Autodesk Inventor part; units mm, degrees
ref_plane "YZ Plane" through (0, 0, 0) normal (1, 0, 0) x (0, 1, 0)
ref_plane "XZ Plane" through (0, 0, 0) normal (0, 1, 0) x (-1, 0, 0)
ref_plane "XY Plane" through (0, 0, 0) normal (0, 0, 1) x (1, 0, 0)
sketch "Sketch1" plane through (0, 0, 0) normal (0, 1, 0) x (-1, 0, 0)
  line L0 (0, 0) -> (25.4, 0)
  line L1 (25.4, 0) -> (25.4, -10)
  line L2 (25.4, -10) -> (0, -10)
  line L3 (0, -10) -> (0, 0)
  line L4 (25.4, -5) -> (19.05, -5)
  line L5 (19.05, -5) -> (6.35, -5)
  dimension "d0" = 25.4
  dimension "d1" = 10
  dimension "d4" = 6.35
  dimension "d5" = 12.7
extrude "Extrusion1" add sketch "Sketch1" along normal blind 4.445
hole "Hole1" at (-6.35, 0, -5) at (-19.05, 0, -5) direction (0, 1, 0) diameter 10.795 depth 3.175
sketch "Sketch2" plane through (0, 0, 0) normal (0, -1, 0) x (1, 0, 0)
  line L0 (-25.4, 0) -> (0, 0)
  line L1 (0, -10) -> (-25.4, -10)
  line L2 (0, 0) -> (-0.635, 0)
  line L3 (-0.635, 0) -> (-0.635, -10)
  line L4 (-0.635, -10) -> (0, -10)
  line L5 (0, -10) -> (0, 0)
  line L6 (-17.017, 0) -> (-8.383, 0)
  line L7 (-12.7, 0) -> (-12.0585, 0)
  line L8 (-12.0585, 0) -> (-12.0585, -10)
  line L9 (-12.0585, -10) -> (-12.7, -10)
  line L10 (-12.7, -10) -> (-12.7, 0)
  line L11 (-12.7, -10) -> (-13.3295, -10)
  line L12 (-13.3295, -10) -> (-13.3295, 0)
  line L13 (-13.3295, 0) -> (-12.7, 0)
  line L14 (-12.7, 0) -> (-12.7, -10)
  line L15 (-25.4, -10) -> (-25.4, 0)
  line L16 (-25.4, 0) -> (-21.083, 0)
  line L17 (-25.4, -10) -> (-24.765, -10)
  line L18 (-24.765, -10) -> (-24.765, 0)
  line L19 (-24.765, 0) -> (-25.4, 0)
  line L20 (-25.4, 0) -> (-25.4, -10)
  point P0 (-24.765, 0)
  dimension "d13" = 0.635
  dimension "d14" = 0.635
sketch "Sketch3" plane through (0, 0, 0) normal (1, 0, 0) x (0, 0, -1)
  line L0 (0, 4.445) -> (10, 4.445)
  line L1 (5, 4.445) -> (9.445, 0)
  line L2 (10, 0) -> (0, 0)
  line L3 (5, 4.445) -> (11.2862, 4.445) construction
  dimension "d15" = 45
extrude "Extrusion2" add sketch "Sketch2" along normal blind 25.4 contours L0 L18 L1 L15 | L12 L0 L10 L1 | L10 L0 L8 L1 | L3 L0 L5 L1
sketch "Sketch4" plane through (0, 4.445, 0) normal (1, 0, 0) x (0, 0, -1)
  line L0 (0, -4.445) -> (10, -14.445)
  line L1 (10, -29.845) -> (10, 0)
  line L2 (0, -4.445) -> (14.1421, -4.445) construction
  line L3 (0, -4.445) -> (0, -29.845)
  line L4 (0, -4.445) -> (0, -29.845)
  line L5 (0, -29.845) -> (10, -29.845)
  line L6 (0, -29.845) -> (10, -29.845)
  line L7 (10, -29.845) -> (10, -14.445)
  dimension "d18" = 45
extrude "Extrusion3" cut sketch "Sketch4" against normal blind 25.4
sketch "Sketch5" plane through (0, 4.445, -10) normal (0, 0, -1) x (-1, 0, 0)
  line L0 (25.4, -14.445) -> (25.4, -4.445)
  line L1 (-13.6769, -18.89) -> (25.4, -18.89)
  line L2 (25.4, -18.89) -> (25.4, -6.19)
  line L3 (25.4, -6.19) -> (-13.6769, -6.19)
  line L4 (-13.6769, -6.19) -> (-13.6769, -18.89)
  line L5 (0, -14.445) -> (0, 0)
  line L6 (0, -6.19) -> (25.4, -6.19)
  line L7 (25.4, -6.19) -> (25.4, -26.51)
  line L8 (25.4, -26.51) -> (0, -26.51)
  line L9 (0, -26.51) -> (0, -6.19)
  point P0 (0, -4.445)
  point P1 (25.4, -18.89)
  dimension "d21" = 12.7
  dimension "d28" = 20.32
extrude "Extrusion4" add sketch "Sketch5" along normal blind 3.175 contours L2 L1 L9 L5 L3 L0 | L7 L8 L9 L1
sketch "Sketch6" plane through (0, 4.445, -13.175) normal (0, 0, -1) x (-1, 0, 0)
  line L0 (12.0585, -6.19) -> (13.3295, -6.19)
  line L1 (12.694, -6.19) -> (12.694, -11.3085)
  line L2 (12.694, -11.3085) -> (12.694, -19.0349)
  line L3 (12.694, -16.1482) -> (7.995, -16.1482)
  line L4 (7.995, -16.1482) -> (17.393, -16.1482)
  line L5 (7.995, -21.2233) -> (7.995, -11.0732) construction
  line L6 (9.265, -21.2233) -> (9.265, -11.0732)
  line L7 (6.725, -11.0732) -> (6.725, -21.2233)
  arc A0 (6.725, -21.2233) -> (9.265, -21.2233) centre (7.995, -21.2233) ccw
  arc A1 (9.265, -11.0732) -> (6.725, -11.0732) centre (7.995, -11.0732) ccw
  line L8 (17.393, -21.2233) -> (17.393, -11.0732) construction
  line L9 (18.663, -21.2233) -> (18.663, -11.0732)
  line L10 (16.123, -11.0732) -> (16.123, -21.2233)
  arc A2 (16.123, -21.2233) -> (18.663, -21.2233) centre (17.393, -21.2233) ccw
  arc A3 (18.663, -11.0732) -> (16.123, -11.0732) centre (17.393, -11.0732) ccw
  line L11 (7.995, -25.0382) -> (7.995, -7.2582) construction
  line L12 (9.265, -25.0382) -> (9.265, -7.2582)
  line L13 (6.725, -7.2582) -> (6.725, -25.0382)
  arc A4 (6.725, -25.0382) -> (9.265, -25.0382) centre (7.995, -25.0382) ccw
  arc A5 (9.265, -7.2582) -> (6.725, -7.2582) centre (7.995, -7.2582) ccw
  line L14 (17.393, -25.0382) -> (17.393, -7.2582) construction
  line L15 (18.663, -25.0382) -> (18.663, -7.2582)
  line L16 (16.123, -7.2582) -> (16.123, -25.0382)
  arc A6 (16.123, -25.0382) -> (18.663, -25.0382) centre (17.393, -25.0382) ccw
  arc A7 (18.663, -7.2582) -> (16.123, -7.2582) centre (17.393, -7.2582) ccw
  point P0 (0, -4.445)
  point P1 (18.663, -11.0732)
  dimension "d24" = 4.699
  dimension "d25" = 9.398
  dimension "d26" = 2.54
  dimension "d27" = 2.54
  dimension "d29" = 8.89
  dimension "d30" = 2.54
  dimension "d31" = 8.89
  dimension "d32" = 2.54
extrude "Extrusion5" cut sketch "Sketch6" against normal blind 3.175
properties part number "door limit switch holder"
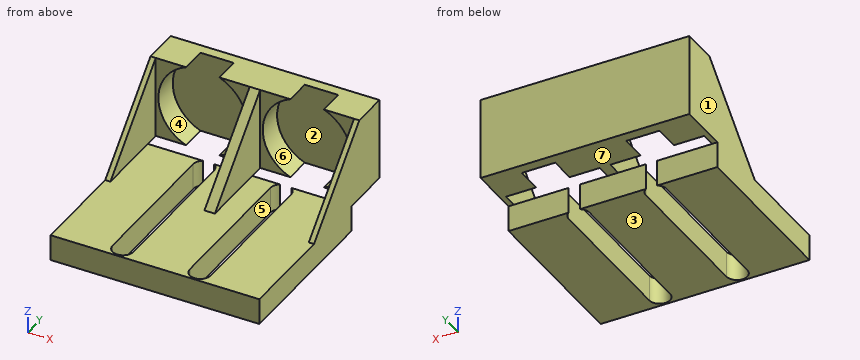
CAD build for the part. Positions are in the model's coordinates, mm. Face numbers are marked on the shaded views. A direction names the side the tool comes from. Round coordinates to 2 decimals unless told otherwise and drop trailing zeros. Write each loop counter-clockwise with the first axis right and the second up, starting at its lowest first coordinate (ties: lowest second). Pieces come first, ordered by that corner, then holes. Notation, with made-up numbers: (86, 20.5) - (90, 20.5) arc R14 cw to (90, 29.5) - close; hole circle Ø7 at (-13.75, 63). An arc over 180 degrees is marked (long way). Return JSON: item names as keys, results as strings. Group by question number.
Item 1: Flat gauge pins, fed straight in: pin 1 Ø1.8 at (x, z) = (-2, -4.5) entering from -Y (3 decimals); pin 2 Ø3 at (x, y) = (-17, 3) entering from -Z; pin 3 Ø1.6 at (y, z) = (-15.5, -11) entering from +X; pin 4 Ø5 at (x, y) = (-20.5, -8.5) entering from +Z. Where does each tip first touch, or does it go through?
Item 2: 3-axis set-ups, long thin cutter, end or side, ignore diameter. For the marked faces 5, 6 and 7: which of +Z, -Z, +X, -X, +Y, -Y reach the whole face in a straight line?
Item 3: Band-saw the part on B-B on y = -12.75. List the corners of the cut face in (x, z) (3 decimals), plus the area to 3 significant figures.
Item 4: Band-saw the part on D-D on y = -8. List the corners of the cut face in (x, z) (1 decimal), plus the area to 3 significant figures.
Item 5: Probe probe 1 along X at (y, z) = (-5, -11) (3 decimals); probe 2 along X at (y, z) = (2.75, -1.5); probe 3 along Z at (x, y) = (-11, -7.5) (3 decimals). List the from-to ranges inside material, lowest first.
Item 6: Band-saw the part on A-A on x = -19.5. List the corners of the cut face in (y, z) (3 decimals), plus the area to 3 significant figures.
Item 7: Mould opens along Z. For the marked faces 1, 2, 3 and 4 say: +Z half, -Z half, draft (parallel to the pull), parting line (faces both ways), or undercut.
Item 8: Band-saw the part on C-C on z = -11.5. List the corners of the cut face in (x, y) (3 decimals), plus the area to 3 significant figures.
Resolved:
{
 "1": {"pin 1": "stops at y = 3.175", "pin 2": "stops at z = -10", "pin 3": "stops at x = 0", "pin 4": "stops at z = -10"},
 "2": {"face 5": "+Z, -Z", "face 6": "-Y", "face 7": "-Z, +X, -X, +Y"},
 "3": {"outline": "(-25.4, -13.175) - (-18.663, -13.175) - (-18.663, -10) - (-25.4, -10) - close; (-16.123, -13.175) - (-9.265, -13.175) - (-9.265, -10) - (-16.123, -10) - close; (-6.725, -13.175) - (0, -13.175) - (0, -10) - (-6.725, -10) - close", "area": "64.5 mm²"},
 "4": {"outline": "(-25.4, -13.2) - (-18.7, -13.2) - (-18.7, -10) - (-24.8, -10) - (-24.8, -8) - (-25.4, -8) - close; (-16.1, -13.2) - (-9.3, -13.2) - (-9.3, -10) - (-12.1, -10) - (-12.1, -8) - (-13.3, -8) - (-13.3, -10) - (-16.1, -10) - close; (-6.7, -13.2) - (0, -13.2) - (0, -8) - (-0.6, -8) - (-0.6, -10) - (-6.7, -10) - close", "area": "69.6 mm²"},
 "5": {"probe 1": "x = -25.4 to -18.663, -16.123 to -9.265, -6.725 to 0", "probe 2": "x = -25.4 to -23.16, -14.94 to -10.46, -2.24 to 0", "probe 3": "z = -13.175 to -10"},
 "6": {"outline": "(-22.065, -13.175) - (-1.745, -13.175) - (-1.745, -10) - (-22.065, -10) - close; (3.175, -10) - (4.445, -10) - (4.445, 0) - (3.175, 0) - close", "area": "77.2 mm²"},
 "7": {"face 1": "draft", "face 2": "undercut", "face 3": "-Z half", "face 4": "undercut"},
 "8": {"outline": "(-25.4, -22.065) - (0, -22.065) - (0, -1.745) - (-7.308, -1.745) arc R1.27 cw to (-6.725, -2.813) - (-6.725, -20.593) arc R1.27 cw to (-9.265, -20.593) - (-9.265, -2.813) arc R1.27 cw to (-8.682, -1.745) - (-16.706, -1.745) arc R1.27 cw to (-16.123, -2.813) - (-16.123, -20.593) arc R1.27 cw to (-18.663, -20.593) - (-18.663, -2.813) arc R1.27 cw to (-18.08, -1.745) - (-25.4, -1.745) - close", "area": "416 mm²"}
}
